The listing builds one solid part. Answer for the finished solid, in the listing's coordinates (mm). A direction names the side the tool comes from. Give positions to 0.01 mm unless a question says otherwise; leave off trailing zeros. Loops run counter-clockwise (first coordinate to the right, second up) from the corner with the lowest first, then second, coordinate; pieces in that order, holes last. Notation, with made-up numbers: (-37, -34) -> (-7, -34) arc R23 cw to (-7, -5) -> close; hole circle Ø9 at (25.25, 6). An arc over 180 degrees is marked (long way). One line per question, with ' | ' between items. Start each with the question number.
from build123d import *

# Parameters (mm, degrees)
SKETCH_1_W          = 398
SKETCH_1_H          = 300
EXTRUDE_1_DEPTH     = 90
FILLET_1_R          = 35
SKETCH_2_R          = 11.25
CUT_EXTRUDE_1_DEPTH = 90
SHELL_1_T           = -2


with BuildPart() as part:
    # 草图1 → 凸台-拉伸1 (new body)
    with BuildSketch(Plane(origin=(0, 0, 0), x_dir=(1, 0, 0), z_dir=(0, 1, 0))):
        Rectangle(SKETCH_1_W, SKETCH_1_H)
    extrude(amount=EXTRUDE_1_DEPTH)

    # 圆角1
    fillet_1_edges = [part.edges().sort_by_distance(p)[0] for p in [
        (199, 45, 150),
        (-199, 45, 150),
        (-199, 45, -150),
        (199, 45, -150),
    ]]
    fillet(fillet_1_edges, radius=FILLET_1_R)

    # 草图2 → 切除-拉伸1 (cut)
    with BuildSketch(Plane(origin=(0, 90, 0), x_dir=(1, 0, 0), z_dir=(0, 1, 0))):
        with Locations((-199, 25.5)):
            Circle(SKETCH_2_R)
        with Locations((-199, -25.5)):
            Circle(SKETCH_2_R)
        with Locations((199, -25.5)):
            Circle(SKETCH_2_R)
        with Locations((199, 25.5)):
            Circle(SKETCH_2_R)
    extrude(amount=-CUT_EXTRUDE_1_DEPTH, mode=Mode.SUBTRACT)

    # 抽壳1
    shell_1_openings = [part.faces().sort_by_distance(p)[0] for p in [
        (0, 90, 0),
    ]]
    offset(amount=SHELL_1_T, openings=shell_1_openings, kind=Kind.INTERSECTION)


solid = part.part
1. Determine the mould class of faces 3 (the cylindrical face through (-189.019, 45.63, 139.475)), 4 (the flat face through (-199, 44, 0)), 5 (the flat face through (-2, 45, -148)), 6 (the cylindrical face through (-187.59, 46.616, 138.077)) for opening direction Z: released by +Z, released by -Z, zero draft, split by the parting line, or undercut.
2. Each of these flat-tipped pins is pushed along its axis until it touches: pin 1 Ø6 at (y, z) = (70.5, 23.5) entering from -X; pin 2 Ø2 at (x, z) = (89, 111) entering from +Y; pin 3 Ø2 at (y, z) = (23.5, -33) entering from -X. Where does it stop, or does it pass through?
3. The part is cut by section C-C (x = -147). Write down the section's boundary in (y, z), plus the area to 3 significant figures.
4. The part is cut by section B-B (z = 78.5). Write down the section's boundary in (x, y), plus the area to 3 significant figures.
5. Straight lines are drawn through the part: L1, parallel to X at y = 25, z = -51; L2, parallel to Z at x = -138, y = 65.5; L3, parallel to X at y = 44, z = -26.5. For each, find the intervals that lie inside material, in ascending order.
6. For faces 1 (the cylindrical face through (187.753, 45.63, 25.253)), 2 (the flat face through (-197, 45, 77)), determine the directions among +Z, -Z, +X, -X, +Y, -Y from which every point of the face is accessible in a straight line to the end or side of a thin tool.
Check sheet entries:
1) face 3: released by +Z | face 4: zero draft | face 5: undercut | face 6: undercut
2) pin 1: stops at x = -188.92 | pin 2: stops at y = 2 | pin 3: stops at x = -191.63
3) outline: (0, -150) -> (90, -150) -> (90, -148) -> (2, -148) -> (2, 148) -> (90, 148) -> (90, 150) -> (0, 150) -> close | area: 952 mm^2
4) outline: (-199, 0) -> (199, 0) -> (199, 90) -> (197, 90) -> (197, 2) -> (-197, 2) -> (-197, 90) -> (-199, 90) -> close | area: 1,150 mm^2
5) L1: x = -199 to -197, 197 to 199 | L2: z = -150 to -148, 148 to 150 | L3: x = -187.79 to -185.79, 185.79 to 187.79
6) face 1: +X, +Y, -Y | face 2: +Y
